```python
from build123d import *

# Parameters (mm, degrees)
SKETCH1_R           = 1.6
BOSS_EXTRUDE1_DEPTH = 6


with BuildPart() as part:
    # Sketch1 → Boss-Extrude1 (new body)
    with BuildSketch(Plane.XY):
        Polygon((-55.855858156, -19), (-55.855858156, -40), (-32.018263016, -40), (-32.018263016, -34), (7.981736984, -34), (7.981736984, -40), (31.819332123, -40), (31.819332123, 27.498322337), (-55.855858156, 27.498322337), (-55.855858156, 11), (-49.855858156, 11), (-49.855858156, -19), align=None)
        with BuildLine():
            ThreePointArc((-26.8550349, -6.369230763), (-27.6, 2.9e-08), (-26.855034887, 6.369230819))
            ThreePointArc((-26.855034887, 6.369230819), (-24.84706156, 12.015969866), (-21.667528577, 17.096145922))
            ThreePointArc((-21.667528577, 17.096145922), (-19.420359041, 17.361153612), (-19.15535135, 15.113984076))
            ThreePointArc((-19.15535135, 15.113984076), (-21.966242856, 10.622813883), (-23.741407682, 5.630769153))
            ThreePointArc((-23.741407682, 5.630769153), (-24.4, 3e-09), (-23.741407684, -5.630769147))
            ThreePointArc((-23.741407684, -5.630769147), (-22.28057337, -9.946660258), (-20.042787404, -13.9156988))
            ThreePointArc((-20.042787404, -13.9156988), (-20.444563705, -16.142484781), (-22.671349686, -15.740708479))
            ThreePointArc((-22.671349686, -15.740708479), (-25.202615761, -11.251140334), (-26.8550349, -6.369230763))
        make_face(mode=Mode.SUBTRACT)
        with Locations((26, 0)):
            Circle(SKETCH1_R, mode=Mode.SUBTRACT)
    extrude(amount=BOSS_EXTRUDE1_DEPTH)


solid = part.part
```
Work out the finished part from the listing and answer in its coordinate system (mm). A direction names the side the tool comes from. Give positions to 0.01 mm unless a question says otherwise; leave off trailing zeros. Order: outer loops, then holes, each group sorted by start corner. A loop starts at its lowest first (then second) coordinate and runs counter-clockwise, first axis right, second up. Notation, with made-up numbers: (9.5, 68) - (17.5, 68) arc R15 cw to (17.5, 94) - close; hole circle Ø1 at (-27.75, 19). An arc over 180 degrees is marked (long way). One line per item, written item: value. Start each with the question number.
1. Consider line 1 (Y direction, x = 26, z = 2.1); line 2 (X direction, y = -36, z = 5.7); line 3 (Y direction, x = -4, z = 1.3). Determine where each line is inside the solid, lowest interval first.
2. For a pull along X with two mould halves and no side action, classify faces 1 (the face through (20, -40, 3)), 2 (the face through (24.82, 1.08, 2.96)), 3 (the face through (-49.856, -4, 3)) as released by +X, released by -X, zero draft, split by the parting line, or undercut.
3. Each of these flat-tipped pins is pushed along its axis until it touches: pin 1 Ø1.8 at (x, z) = (-17, 4) entering from -Y; pin 2 Ø1.8 at (y, z) = (-3.5, 3) entering from -X. Where does it stop, or does it pass through?
4. Section D-D, the plane y = 9 is taken. Write down the section's boundary in (x, z).
5. Section C-C, the plane x = 26 is taken. Write down the section's boundary in (y, z), then the cut area to 3 significant figures.
6. Section B-B, the plane y = 0 is taken. Write down the section's boundary in (x, z), then the cut area to 3 significant figures.
7. Section A-A, the plane z = 4.5 is taken. Write down the section's boundary in (x, y).
8. Which of the six approach directions +Z, -Z, +X, -X, +Y, -Y give full straight-line access (tool end or side, diameter ignored) to faces 4 (the face through (7.982, -37, 3)), 5 (the face through (-53, -19, 3)), 6 (the face through (-19.448, 17.383, 2.958))?
Filled sheet:
1. line 1: -40 to -1.6, 1.6 to 27.5
1. line 2: -55.86 to -32.02, 7.98 to 31.82
1. line 3: -34 to 27.5
2. face 1: zero draft
2. face 2: undercut
2. face 3: released by -X
3. pin 1: y = -34
3. pin 2: x = -49.86
4. outline: (-49.86, 0) - (-26.09, 0) - (-26.09, 6) - (-49.86, 6) - close; (-22.68, 0) - (31.82, 0) - (31.82, 6) - (-22.68, 6) - close
5. outline: (-40, 0) - (-1.6, 0) - (-1.6, 6) - (-40, 6) - close; (1.6, 0) - (27.5, 0) - (27.5, 6) - (1.6, 6) - close
5. area: 386 mm²
6. outline: (-49.86, 0) - (-27.6, 0) - (-27.6, 6) - (-49.86, 6) - close; (-24.4, 0) - (24.4, 0) - (24.4, 6) - (-24.4, 6) - close; (27.6, 0) - (31.82, 0) - (31.82, 6) - (27.6, 6) - close
6. area: 452 mm²
7. outline: (-55.86, -40) - (-32.02, -40) - (-32.02, -34) - (7.98, -34) - (7.98, -40) - (31.82, -40) - (31.82, 27.5) - (-55.86, 27.5) - (-55.86, 11) - (-49.86, 11) - (-49.86, -19) - (-55.86, -19) - close; hole (-22.67, -15.74) arc R1.6 ccw to (-20.04, -13.92) arc R24.4 cw to (-19.16, 15.11) arc R1.6 ccw to (-21.67, 17.1) arc R27.6 ccw to start; hole circle Ø3.2 at (26, 0)
8. face 4: +Z, -Z, -Y
8. face 5: +Z, -Z, -X
8. face 6: +Z, -Z
